Source: CAD feature listing. Evaluate the final solid. Frame: model axes, mm. A direction names the side the tool comes from. Give positions to 0.01 mm unless a question says otherwise; leave off trailing zeros. Write each loop counter-clockwise with the first axis right and the second up, starting at its lowest first coordinate (ties: lowest second). Pieces come first, ordered by that corner, then holes.
```python
from build123d import *

# Parameters (mm, degrees)
SKETCH1_W           = 110
SKETCH1_H           = 80
BOSS_EXTRUDE1_DEPTH = 2
SKETCH2_R           = 1.6
CUT_EXTRUDE1_DEPTH  = 3
SKETCH3_W           = 34.042558981
SKETCH3_H           = 11.036345557
CUT_EXTRUDE2_DEPTH  = 3
SKETCH4_W           = 2
SKETCH4_H           = 68.963654443
BOSS_EXTRUDE2_DEPTH = 3
SKETCH5_W           = 75.957441019
SKETCH5_H           = 2
BOSS_EXTRUDE3_DEPTH = 1
SKETCH6_W           = 113
SKETCH6_H           = 3
BOSS_EXTRUDE4_DEPTH = 2.2
SKETCH7_W           = 113
SKETCH7_H           = 13
BOSS_EXTRUDE6_DEPTH = 2
SKETCH10_W          = 37.04
SKETCH10_H          = 81
CUT_EXTRUDE5_DEPTH  = 3
SKETCH10_2_W        = 37.04
SKETCH10_2_H        = 81
CUT_EXTRUDE6_DEPTH  = 2.2
SKETCH12_W          = 25.96
SKETCH12_H          = 81
CUT_EXTRUDE7_DEPTH  = 4.2
SKETCH13_W          = 4.352914054
SKETCH13_H          = 137.927308885
CUT_EXTRUDE8_DEPTH  = 3


with BuildPart() as part:
    # Sketch1 → Boss-Extrude1 (new body)
    with BuildSketch(Plane.XY):
        Rectangle(SKETCH1_W, SKETCH1_H)
    extrude(amount=BOSS_EXTRUDE1_DEPTH)

    # Sketch2 → Cut-Extrude1 (cut, through all)
    with BuildSketch(Plane(origin=(0, 0, 0), x_dir=(-1, 0, 0), z_dir=(0, 0, -1))):
        with Locations((35.470952311, 24.181556833)):
            Circle(SKETCH2_R)
        with Locations((-39.411047689, 24.181556833)):
            Circle(SKETCH2_R)
        with Locations((-45.738047689, -24.040443167)):
            Circle(SKETCH2_R)
        with Locations((36.740952311, -24.040443167)):
            Circle(SKETCH2_R)
    extrude(amount=-CUT_EXTRUDE1_DEPTH, mode=Mode.SUBTRACT)

    # Sketch3 → Cut-Extrude2 (cut, through all)
    with BuildSketch(Plane.XY.offset(2)):
        with Locations((-37.97872051, 34.481827221)):
            Rectangle(SKETCH3_W, SKETCH3_H)
    extrude(amount=-CUT_EXTRUDE2_DEPTH, mode=Mode.SUBTRACT)

    # Sketch4 → Boss-Extrude2 (add)
    with BuildSketch(Plane.ZY.offset(55)):
        with Locations((1, -5.518172778)):
            Rectangle(SKETCH4_W, SKETCH4_H)
    extrude(amount=BOSS_EXTRUDE2_DEPTH)

    # Sketch5 → Boss-Extrude3 (add)
    with BuildSketch(Plane(origin=(0, 40, 0), x_dir=(1, 0, 0), z_dir=(0, 1, 0))):
        with Locations((17.02127949, -1)):
            Rectangle(SKETCH5_W, SKETCH5_H)
    extrude(amount=BOSS_EXTRUDE3_DEPTH)

    # Sketch6 → Boss-Extrude4 (add)
    with BuildSketch(Plane(origin=(0, 0, 0), x_dir=(-1, 0, 0), z_dir=(0, 0, -1))):
        with Locations((1.5, 29.5)):
            Rectangle(SKETCH6_W, SKETCH6_H)
        with Locations((1.5, -28.5)):
            Rectangle(SKETCH6_W, SKETCH6_H)
    extrude(amount=BOSS_EXTRUDE4_DEPTH)

    # Sketch7 → Boss-Extrude6 (add)
    with BuildSketch(Plane(origin=(0, 0, -2.2), x_dir=(-1, 0, 0), z_dir=(0, 0, -1))):
        with Locations((1.5, 34.5)):
            Rectangle(SKETCH7_W, SKETCH7_H)
        with Locations((1.5, -33.5)):
            Rectangle(SKETCH7_W, SKETCH7_H)
    extrude(amount=BOSS_EXTRUDE6_DEPTH)

    # Sketch10 → Cut-Extrude5 (cut, through all)
    with BuildSketch(Plane.XY.offset(-2.2)):
        with Locations((-39.48, 0.5)):
            Rectangle(SKETCH10_W, SKETCH10_H)
    extrude(amount=-CUT_EXTRUDE5_DEPTH, mode=Mode.SUBTRACT)

    # Sketch10<2> → Cut-Extrude6 (cut)
    with BuildSketch(Plane.XY.offset(-2.2)):
        with Locations((-39.48, 0.5)):
            Rectangle(SKETCH10_2_W, SKETCH10_2_H)
    extrude(amount=CUT_EXTRUDE6_DEPTH, mode=Mode.SUBTRACT)

    # Sketch12 → Cut-Extrude7 (cut)
    with BuildSketch(Plane(origin=(0, 0, -4.2), x_dir=(-1, 0, 0), z_dir=(0, 0, -1))):
        with Locations((-19.02, 0.5)):
            Rectangle(SKETCH12_W, SKETCH12_H)
    extrude(amount=-CUT_EXTRUDE7_DEPTH, mode=Mode.SUBTRACT)

    # Sketch13 → Cut-Extrude8 (cut, through all)
    with BuildSketch(Plane(origin=(0, 0, 0), x_dir=(-1, 0, 0), z_dir=(0, 0, -1))):
        with Locations((58, 28.963654443)):
            Rectangle(SKETCH13_W, SKETCH13_H)
    extrude(amount=-CUT_EXTRUDE8_DEPTH, mode=Mode.SUBTRACT)


solid = part.part
```
1. Section query D-D (x = 16.5). Return loops of the section in (y, z).
2. Section query A-A (x = -18.5). Return loops of the section in (y, z).
3. Pin query (flat end, axial travel): P1, Ø0.7, axis at x = -10, z = -1.5, coming from the -Y side; P2, Ø2, axis at y = 36.5, z = -2.5, coming from the -X side; P3, Ø5, axis at x = 9, y = 6.5, coming from the -Z side. Return the tip coordinate at first contact, or that it passes through.
4. Access query for faces 1 (the flat face through (44, 28, -2)), 2 (the flat face through (32, 33, -3)), 3 (the flat face through (-20.96, 33, -3)), 4 (the flat face through (-7, 31, -1)). Directions: +Z, -Z, +X, -X, +Y, -Y. A direction counts if a zero-diameter tool reaches every point of the face in a straight line with its end or side. Return the directions, or none.
5. Section query B-B (z = 1). Return loops of the section in (x, y).
6. Section query C-C (y = 11.5). Return loops of the section in (x, z).
7. Line query: probe 1 along Y at (x, z) = (44, -0.5); probe 2 along X at (y, z) = (-29, -1); probe 3 along Z at (x, y) = (48, -32). Output: solid intervals per line, ascending.
8. Pull-direction query (Z, two-part tool) for faces 5 (the flat face through (-20.96, -32, -3)), 6 (the flat face through (-1, 0, 2)), 7 (the flat face through (44, -35, -2.2)); classes: pulls with the +Z half, pulls with the -Z half, needs draft (parallel to the pull), parting line crosses it, or undercut.
The answers:
1. outline: (-40, 0) - (41, 0) - (41, 2) - (-40, 2) - close
2. outline: (-40, -4.2) - (-27, -4.2) - (-27, 0) - (28, 0) - (28, -4.2) - (41, -4.2) - (41, -2.2) - (31, -2.2) - (31, 0) - (41, 0) - (41, 2) - (-40, 2) - (-40, 0) - (-30, 0) - (-30, -2.2) - (-40, -2.2) - close
3. P1: stops at y = -30
3. P2: stops at x = -20.96
3. P3: stops at z = 0
4. face 1: -Z, +X, -X
4. face 2: -Z, +Y, -Y
4. face 3: -Z, -X, +Y, -Y
4. face 4: +X, -X, +Y
5. outline: (-55.82, -40) - (55, -40) - (55, 41) - (-20.96, 41) - (-20.96, 28.96) - (-55.82, 28.96) - close; hole circle Ø3.2 at (-36.74, -24.04); hole circle Ø3.2 at (-35.47, 24.18); hole circle Ø3.2 at (39.41, 24.18); hole circle Ø3.2 at (45.74, -24.04)
6. outline: (-55.82, 0) - (55, 0) - (55, 2) - (-55.82, 2) - close
7. probe 1: y = -30 to -27, 28 to 31
7. probe 2: x = -20.96 to 6.04, 32 to 55
7. probe 3: z = -4.2 to -2.2, 0 to 2
8. face 5: needs draft
8. face 6: pulls with the +Z half
8. face 7: undercut
